Job drawing, mm, ordinate dimensions from the low corner. One solid piece. A direction names the side the tool comes from. Round coordinates to 2 decimals unless told otherwise and drop trailing zeros. Loops run counter-clockwise (first coordinate to the right, second up) from the corner with the lowest first, then second, coordinate; pieces in that order, holes last. Notation, with made-up numbers: M 42.25,72 L 74.25,72 A16 cw 74.25,76 Z; hole C -25,11 d9. An arc over 180 degrees is marked long. Use a Markdown table: item, result. Add a question column.
(1) Band-saw the part on C-C, the plane y = 24.5. Write the cut outline in (x, z).
(2) Flat gauge pins, fed straight in: P1, Ø9, axis at x = 9.5, z = 6.5, coming from the -Y side; P2, Ø3, axis at y = 24.5, z = 13, coming from the +X side; P3, Ø3, axis at x = 16, z = 12.5, coming from the +Y side; P4, Ø8, axis at x = 10.5, y = 38.5, coming from the -Z side. Where does each tip first touch, or does it go through?
(3) Band-saw the part on B-B, the plane x = 9. Write the cut outline in (y, z).
(4) Band-saw the part on A-A, the plane z = 9. Write the cut outline in (x, y).
(5) Two-plate mould, pull along Y, no slides. Class the marked faces 1, 2, 3 and 4: released by +Y, released by -Y, zero draft, split by the parting line, or undercut.
(6) Wall check: L1, parallel to Y at x = 9.75, z = 4.75; L2, parallel to Y at x = 7.75, z = 17.25; L3, parallel to Y at x = 10.5, z = 3.5. Give the ranges that are in metal, low to high.
(7) Which spindle directions (+Z, -Z, +X, -X, +Y, -Y) get a long thin tool onto all of the face, cutting with end or side? Do the marked faces 5, 6 and 7. Say none if no direction does.
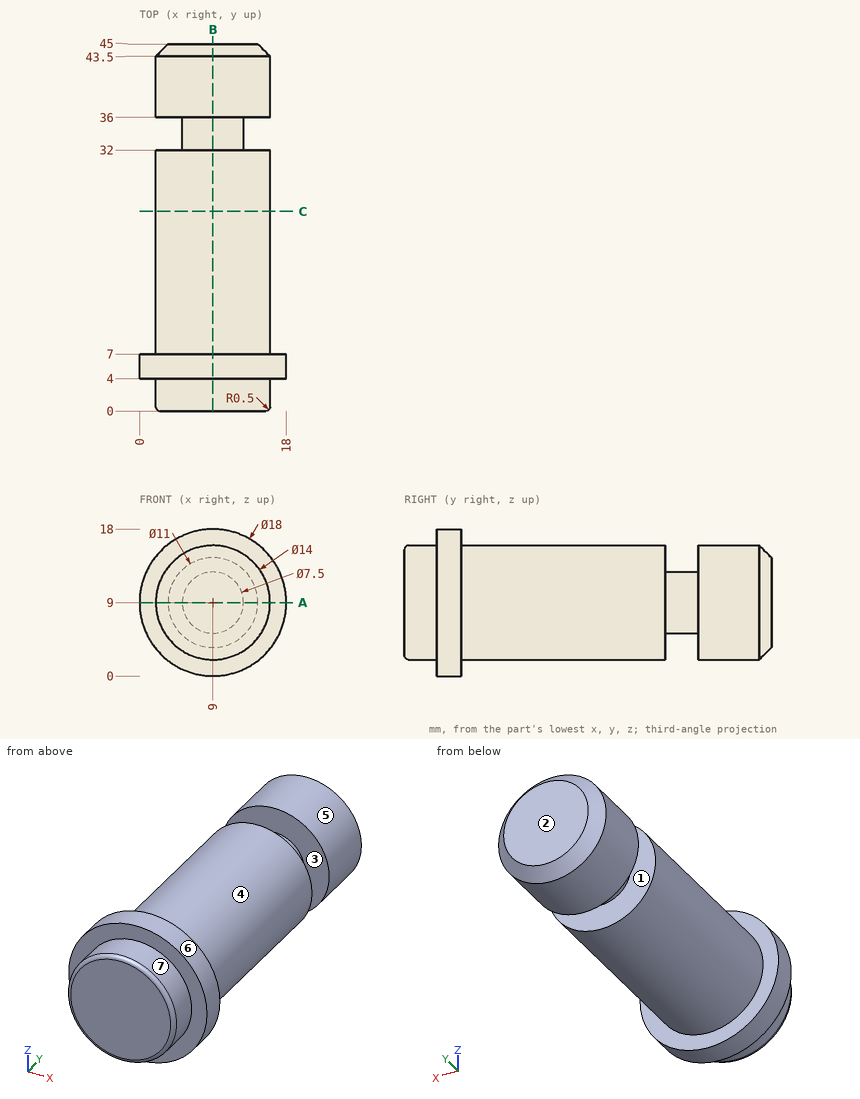
Return value:
| question | item | result |
|---|---|---|
| 1 | outline | C 9,9 d14 |
| 2 | P1 | y = 0 |
| 2 | P2 | x = 15.54 |
| 2 | P3 | y = 44.17 |
| 2 | P4 | z = 2 |
| 3 | outline | M 0,2.5 A0.5 ccw 0.5,2 L 4,2 L 4,0 L 7,0 L 7,2 L 32,2 L 32,5.25 L 36,5.25 L 36,2 L 43.5,2 L 45,3.5 L 45,14.5 L 43.5,16 L 36,16 L 36,12.75 L 32,12.75 L 32,16 L 7,16 L 7,18 L 4,18 L 4,16 L 0.5,16 A0.5 ccw 0,15.5 Z |
| 4 | outline | M 0,4 L 2,4 L 2,0.5 A0.5 ccw 2.5,0 L 15.5,0 A0.5 ccw 16,0.5 L 16,4 L 18,4 L 18,7 L 16,7 L 16,32 L 12.75,32 L 12.75,36 L 16,36 L 16,43.5 L 14.5,45 L 3.5,45 L 2,43.5 L 2,36 L 5.25,36 L 5.25,32 L 2,32 L 2,7 L 0,7 Z |
| 5 | face 1 | undercut |
| 5 | face 2 | released by +Y |
| 5 | face 3 | undercut |
| 5 | face 4 | zero draft |
| 6 | L1 | 0 to 32, 36 to 45 |
| 6 | L2 | 4 to 7 |
| 6 | L3 | 0 to 32, 36 to 44.8 |
| 7 | face 5 | +Y |
| 7 | face 6 | +Y, -Y |
| 7 | face 7 | -Y |
